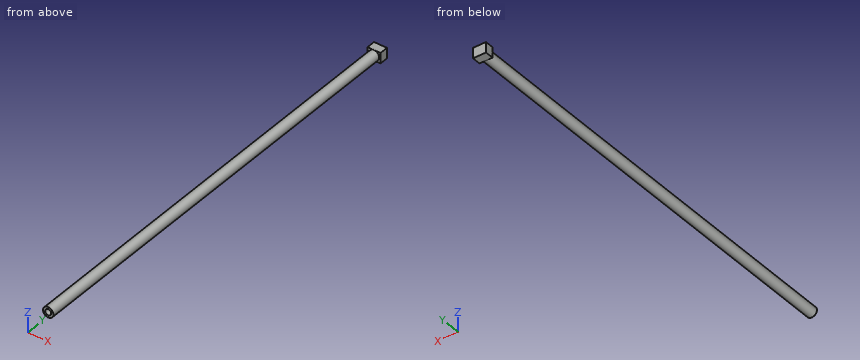
from build123d import *

# Parameters (mm, degrees)
SKETCH_2_R      = 1.2
SKETCH_2_R_2    = 0.7
EXTRUDE_1_DEPTH = 100
SKETCH_3_W      = 3
SKETCH_3_H      = 2.4
EXTRUDE_2_DEPTH = 2


with BuildPart() as part:
    # 草图2 → 凸台-拉伸1 (new body)
    with BuildSketch(Plane(origin=(0, 0, 0), x_dir=(1, 0, 0), z_dir=(0, 1, 0))):
        with Locations(Location((0, 0, 0), (0, 0, 270))):
            Circle(SKETCH_2_R)
        with Locations(Location((0, 0, 0), (0, 0, 270))):
            Circle(SKETCH_2_R_2, mode=Mode.SUBTRACT)
    extrude(amount=EXTRUDE_1_DEPTH)

    # 草图3 → 凸台-拉伸2 (add)
    with BuildSketch(Plane(origin=(0, 100, 0), x_dir=(1, 0, 0), z_dir=(0, 1, 0))):
        Rectangle(SKETCH_3_W, SKETCH_3_H)
    extrude(amount=EXTRUDE_2_DEPTH)


solid = part.part
Verification items for the finished model (mm, model axes). Coordinates: 2 decimals unless noted, no trailing zeros. Order: outer loops, then holes, each group sorted by start corner. A loop starts at its lowest first (then second) coordinate and runs counter-clockwise, first axis right, second up. Notation, with made-up numbers: M 30.25,70 L 45.25,70 A11 cw 45.25,80 Z; hole C 55,4 d6. An arc over 180 degrees is marked long. One line per item, written item: value. Start each with the question number.
Item 1: Thickness scan on probe 1 along X at (y, z) = (56, 0); probe 2 along Y at (x, z) = (1.25, 0.7); probe 3 along Z at (x, y) = (0.6, 83.5). Record the ranges inside material, lowest first.
Item 2: Sectioned sample at B-B on y = 19. Record the cut outline in (x, z).
Item 3: Depth check by flat-ended pin: P1, Ø1, axis at x = -1, y = 70.5, coming from the +Z side; P2, Ø0.8, axis at x = 0, z = 0, coming from the -Y side; P3, Ø1, axis at x = -1, y = 84.5, coming from the -Z side. Enter the tip coordinate at first touch or a pass-through.
Item 4: Sectioned sample at A-A on z = 0. Record the cut outline in (x, y), then the cut area to 3 significant figures.
Calculated:
1. probe 1: -1.2 to -0.7, 0.7 to 1.2
1. probe 2: 100 to 102
1. probe 3: -1.04 to -0.36, 0.36 to 1.04
2. outline: C 0,0 d2.4; hole C 0,0 d1.4
3. P1: z = 1.09
3. P2: y = 100
3. P3: z = -1.09
4. outline: M -1.5,100 L -1.2,100 L -1.2,0 L -0.7,0 L -0.7,100 L 0.7,100 L 0.7,0 L 1.2,0 L 1.2,100 L 1.5,100 L 1.5,102 L -1.5,102 Z
4. area: 106 mm^2
